Geometry check sheet. Reference: the model listing, model coordinates, mm. A direction names the side the tool comes from. Give positions to 0.01 mm unless a question says otherwise; leave off trailing zeros. Loops run counter-clockwise (first coordinate to the right, second up) from the corner with the lowest first, then second, coordinate; pieces in that order, holes last. Notation, with made-up numbers: (-0.5, 44) - (6.5, 44) arc R36 ccw to (6.5, 79) - close; hole circle Ø3 at (25.25, 84.25). An arc over 180 degrees is marked (long way). One line per question, with ' | ' between items. Start each with the question number.
from build123d import *

# Parameters (mm, degrees)
BOSS_EXTRUDE1_DEPTH = 6.35
SKETCH3_R           = 14.2875
SKETCH3_R_2         = 2.032
CUT_EXTRUDE1_DEPTH  = 6.35


with BuildPart() as part:
    # Sketch2 → Boss-Extrude1 (new body)
    with BuildSketch(Plane.XY):
        Polygon((-125.79203122, -159.641560721), (-74.99203122, -159.641560721), (-68.64203122, -159.641560721), (-68.64203122, -108.841560721), (-74.99203122, -108.841560721), (-74.99203122, -19.941560721), (-125.79203122, -19.941560721), align=None)
    extrude(amount=BOSS_EXTRUDE1_DEPTH)

    # Sketch3 → Cut-Extrude1 (cut)
    with BuildSketch(Plane.XY.offset(6.35)):
        with Locations((-100.39203122, -45.351567892)):
            Circle(SKETCH3_R)
        with Locations((-87.69203122, -146.941560721)):
            Circle(SKETCH3_R_2)
        with Locations((-113.09203122, -146.941560721)):
            Circle(SKETCH3_R_2)
        with Locations((-100.39203122, -146.941560721)):
            Circle(SKETCH3_R_2)
        with Locations((-74.99203122, -146.941560721)):
            Circle(SKETCH3_R_2)
        with Locations((-113.09203122, -121.541560721)):
            Circle(SKETCH3_R_2)
        with Locations((-87.69203122, -121.541560721)):
            Circle(SKETCH3_R_2)
        with Locations((-74.99203122, -121.541560721)):
            Circle(SKETCH3_R_2)
        with Locations((-100.39203122, -121.541560721)):
            Circle(SKETCH3_R_2)
    extrude(amount=-CUT_EXTRUDE1_DEPTH, mode=Mode.SUBTRACT)


solid = part.part
(1) Mould release check, pull along Y, two halves, no side actions. Record for faces 1 (the face through (-100, -19.942, 3)), 2 (the face through (-98, -89, 0)), 3 (the face through (-98.454, -120.931, 3.219)): pulls with the +Y half, pulls with the -Y half, needs draft (parallel to the pull), parting line crosses it, or undercut.
(2) Section check C-C, the plane y = -34. Record the boundary of the cut face in (x, z), and give its area (3 significant figures).
(3) Section check D-D, the plane y = -106.5. Record the boundary of the cut face in (x, z).
(4) Material ranges on line 1 (Y direction, x = -76.5, z = 3.5); line 2 (X direction, y = -66, z = 1.25); line 3 (Y direction, x = -101.5, z = 2.25), recorded low to high.
(5) Section check B-B, the plane z = 4.75. Count the separate pieces of the cut face and the enclosed holes in it, and give its area (3 significant figures).
(6) Section check A-A, the plane x = -104.5. Record the boundary of the cut face in (y, z), and give its area (3 significant figures).
(7) Depth check by flat-ended pin: pin 1 Ø5.5 at (x, y) = (-87.69, -121.54) entering from +Z; pin 2 Ø2 at (y, z) = (-104, 4) entering from +X; pin 3 Ø3 at (x, z) = (-70.5, 2) entering from +Y. Enter the tip coordinate at first touch or a pass-through.
(8) Tool access check on faces 4 (the face through (-76.49, -120.17, 3.22)), 5 (the face through (-74.992, -65, 3)). Record the directions out of +Z, -Z, +X, -X, +Y, -Y that give a thin tool (end or side, any length) a straight path to the whole face; none if there is none.
Numbers:
1) face 1: pulls with the +Y half | face 2: needs draft | face 3: undercut
2) outline: (-125.79, 0) - (-109.07, 0) - (-109.07, 6.35) - (-125.79, 6.35) - close; (-91.72, 0) - (-74.99, 0) - (-74.99, 6.35) - (-91.72, 6.35) - close | area: 212 mm^2
3) outline: (-125.79, 0) - (-74.99, 0) - (-74.99, 6.35) - (-125.79, 6.35) - close
4) line 1: -159.64 to -148.3, -145.58 to -122.9, -120.18 to -19.94 | line 2: -125.79 to -74.99 | line 3: -159.64 to -148.64, -145.24 to -123.24, -119.84 to -59.6, -31.11 to -19.94
5) separate pieces: 1 | enclosed holes: 9 | area: 6,670 mm^2
6) outline: (-159.64, 0) - (-59.04, 0) - (-59.04, 6.35) - (-159.64, 6.35) - close; (-31.67, 0) - (-19.94, 0) - (-19.94, 6.35) - (-31.67, 6.35) - close | area: 713 mm^2
7) pin 1: z = 6.35 | pin 2: x = -74.99 | pin 3: y = -108.84
8) face 4: +Z, -Z | face 5: +Z, -Z, +X, +Y
